```python
from build123d import *

# Parameters (mm, degrees)
SKETCH1_R           = 4.445
BOSS_EXTRUDE1_DEPTH = 3.175


with BuildPart() as part:
    # Sketch1 → Boss-Extrude1 (new body)
    with BuildSketch(Plane(origin=(0, 0, 0), x_dir=(1, 0, 0), z_dir=(0, 1, 0))):
        with BuildLine():
            Line((-27.551576941, 20.997814364), (-41.546014614, 31.663360114))
            ThreePointArc((-41.546014614, 31.663360114), (-42.160017959, 32.737521423), (-41.816542083, 33.926153808))
            ThreePointArc((-41.816542083, 33.926153808), (46.633735943, -26.924), (-50.289182092, 19.251110838))
            ThreePointArc((-50.289182092, 19.251110838), (-49.431534188, 20.142885865), (-48.194281535, 20.148224024))
            Line((-48.194281535, 20.148224024), (-31.960429133, 13.361458364))
            ThreePointArc((-31.960429133, 13.361458364), (-26.396454307, 15.24), (-27.551576941, 20.997814364))
        make_face()
        with Locations(Location((0, 36.5125, 0), (0, 0, 270))):
            Circle(SKETCH1_R, mode=Mode.SUBTRACT)
        with Locations(Location((0, -36.5125, 0), (0, 0, 270))):
            Circle(SKETCH1_R, mode=Mode.SUBTRACT)
        with Locations(Location((30.245937227, -17.4625, 0), (0, 0, 270))):
            Circle(SKETCH1_R, mode=Mode.SUBTRACT)
        with Locations(Location((30.245937227, 17.4625, 0), (0, 0, 270))):
            Circle(SKETCH1_R, mode=Mode.SUBTRACT)
        with Locations(Location((-30.245937227, -17.4625, 0), (0, 0, 270))):
            Circle(SKETCH1_R, mode=Mode.SUBTRACT)
        with BuildLine():
            ThreePointArc((-25.640504728, -5.80310592), (0, -26.289), (25.640504728, -5.80310592))
            ThreePointArc((25.640504728, -5.80310592), (26.904017035, -4.591795724), (28.513791893, -5.279080705))
            ThreePointArc((28.513791893, -5.279080705), (46.0962375, 0), (28.513791893, 5.279080705))
            ThreePointArc((28.513791893, 5.279080705), (26.904017035, 4.591795724), (25.640504728, 5.80310592))
            ThreePointArc((25.640504728, 5.80310592), (0, 26.289), (-25.640504728, 5.80310592))
            ThreePointArc((-25.640504728, 5.80310592), (-26.904017035, 4.591795724), (-28.513791893, 5.279080705))
            ThreePointArc((-28.513791893, 5.279080705), (-46.0962375, 0), (-28.513791893, -5.279080705))
            ThreePointArc((-28.513791893, -5.279080705), (-26.904017035, -4.591795724), (-25.640504728, -5.80310592))
        make_face(mode=Mode.SUBTRACT)
    extrude(amount=BOSS_EXTRUDE1_DEPTH)


solid = part.part
```
The listing builds one solid part. Answer for the finished solid, in the listing's coordinates (mm). A direction names the side the tool comes from. Give positions to 0.01 mm unless a question says otherwise; leave off trailing zeros. Order: outer loops, then holes, each group sorted by start corner. A loop starts at its lowest first (then second) coordinate and runs counter-clockwise, first axis right, second up. Notation, with made-up numbers: (86.25, 14.5) - (98.25, 14.5) arc R22 ccw to (98.25, 22.5) - close; hole circle Ø10 at (-18.75, 32). An arc over 180 degrees is marked (long way). Use one line per item in the form item = value. Start each with the question number.
(1) For faces 1 (the flat face through (12.7, 0, 23.2)), 2 (the cylindrical face through (-26.93, 1.565, 4.587)), 3 (the flat face through (-34.451, 1.565, -26.256)), determine the directions among +Z, -Z, +X, -X, +Y, -Y from which every point of the face is accessible in a straight line to the end or side of a thin tool.
(2) The mould has two halves that part along Z. Classify faces 4 (the cylindrical face through (47.72, 1.57, 24.95)), 5 (the flat face through (12.7, 3.175, 23.2)), 6 (the cylindrical face through (0.2, 1.57, 32.07)): released by +Z, released by -Z, zero draft, split by the parting line, or undercut.
(3) Flat-ended cylindrical pins translate along their axes: pin 1 Ø14 at (x, z) = (0, -36.51) entering from +Y (3 decimals); pin 2 Ø15.5 at (x, z) = (-36.51, 0) entering from +Y; pin 3 Ø1.5 at (y, z) = (2, -40) entering from -X. Find the tip coordinate at first contact, or state that the pin passes through.
(4) A cutting plane is placed at B-B, the plane x = 0. Write down the section's boundary in (y, z) (1 decimal).
(5) A cutting plane is placed at A-A, the plane z = 0. Write down the section's boundary in (x, y) (3 decimals), then the cut area to 3 significant figures.
(6) A cutting plane is placed at D-D, the plane z = 25. Write down the section's boundary in (x, y) (3 decimals), then the cut area to 3 significant figures.
(7) A cutting plane is placed at C-C, the plane y = 0.6. Write down the section's boundary in (x, z) (1 decimal).
(8) Consider line 1 (X direction, y = 1.15, z = -20); line 2 (Z direction, x = -39, y = 2.35); line 3 (Z direction, x = -1, y = 1.9). Determine where each line is inside the solid, lowest interval first. Write a range as from..to.
Ans:
q1.face_1 = +Z, -Z, +X, -X, -Y
q1.face_2 = +Y, -Y
q1.face_3 = -X, +Y, -Y
q2.face_4 = split by the parting line
q2.face_5 = zero draft
q2.face_6 = undercut
q3.pin_1 = 3.175
q3.pin_2 = through
q3.pin_3 = -36.87
q4.outline = (0, -53.8) - (3.2, -53.8) - (3.2, -41) - (0, -41) - close; (0, -32.1) - (3.2, -32.1) - (3.2, -26.3) - (0, -26.3) - close; (0, 26.3) - (3.2, 26.3) - (3.2, 32.1) - (0, 32.1) - close; (0, 41) - (3.2, 41) - (3.2, 53.8) - (0, 53.8) - close
q5.outline = (-53.848, 0) - (-46.096, 0) - (-46.096, 3.175) - (-53.848, 3.175) - close; (46.096, 0) - (53.848, 0) - (53.848, 3.175) - (46.096, 3.175) - close
q5.area = 49.2 mm^2
q6.outline = (-47.693, 0) - (-8.131, 0) - (-8.131, 3.175) - (-47.693, 3.175) - close; (8.131, 0) - (47.693, 0) - (47.693, 3.175) - (8.131, 3.175) - close
q6.area = 251 mm^2
q7.outline = (-50.3, -19.3) arc R1.6 ccw to (-48.2, -20.1) - (-32, -13.4) arc R4.4 cw to (-27.6, -21) - (-41.5, -31.7) arc R1.6 ccw to (-41.8, -33.9) arc R53.8 ccw (long way) to start; hole circle Ø8.9 at (-30.2, 17.5); hole (-28.5, -5.3) arc R1.6 cw to (-25.6, -5.8) arc R26.3 ccw to (25.6, -5.8) arc R1.6 cw to (28.5, -5.3) arc R9.6 ccw (long way) to (28.5, 5.3) arc R1.6 cw to (25.6, 5.8) arc R26.3 ccw to (-25.6, 5.8) arc R1.6 cw to (-28.5, 5.3) arc R9.6 ccw (long way) to start; hole circle Ø8.9 at (0, -36.5); hole circle Ø8.9 at (0, 36.5); hole circle Ø8.9 at (30.2, -17.5); hole circle Ø8.9 at (30.2, 17.5)
q8.line_1 = -49.69..-47.84, -26.6..-17.06, 17.06..26.6, 33.9..50
q8.line_2 = -37.13..-29.72, -16.3..-9.26, 9.26..37.13
q8.line_3 = -53.84..-40.84, -32.18..-26.27, 26.27..32.18, 40.84..53.84
